```python
from build123d import *

# Parameters (mm, degrees)
SKETCH1_W           = 34.4
SKETCH1_H           = 36
BOSS_EXTRUDE1_DEPTH = 5
SKETCH4_R           = 1.5
CUT_EXTRUDE2_DEPTH  = 5
SKETCH4_3_R         = 1.5
SKETCH4_3_W         = 25.4
SKETCH4_3_H         = 25.4
CUT_EXTRUDE3_DEPTH  = 26.393700006
SKETCH7_W           = 5
SKETCH7_H           = 12
CUT_EXTRUDE4_DEPTH  = 5
SKETCH8_W           = 15
SKETCH8_H           = 3
CUT_EXTRUDE5_DEPTH  = 26.393700006
SKETCH9_W           = 6.4
SKETCH9_H           = 3
CUT_EXTRUDE6_DEPTH  = 26.393700006
SKETCH10_W          = 2
SKETCH10_H          = 3
CUT_EXTRUDE7_DEPTH  = 26.393700006
SKETCH11_W          = 2
SKETCH11_H          = 3
SKETCH11_W_2        = 15
CUT_EXTRUDE8_DEPTH  = 26.393700006
SKETCH12_W          = 5
SKETCH12_H          = 16.7
CUT_EXTRUDE9_DEPTH  = 26.393700006
SKETCH13_W          = 2
SKETCH13_H          = 3
CUT_EXTRUDE10_DEPTH = 26.393700006


with BuildPart() as part:
    # Sketch1 → Boss-Extrude1 (new body)
    with BuildSketch(Plane(origin=(0, 0, 0), x_dir=(1, 0, 0), z_dir=(0, 1, 0))):
        Rectangle(SKETCH1_W, SKETCH1_H)
    extrude(amount=BOSS_EXTRUDE1_DEPTH)

    # Sketch4 → Cut-Extrude2 (cut)
    with BuildSketch(Plane(origin=(0, 5, 0), x_dir=(1, 0, 0), z_dir=(0, 1, 0))):
        with Locations(Location((-12.7, 15.5, 0), (0, 0, 270))):
            Circle(SKETCH4_R)
    extrude(amount=-CUT_EXTRUDE2_DEPTH, mode=Mode.SUBTRACT)

    # Sketch4_3 → Cut-Extrude3 (cut, through all)
    with BuildSketch(Plane(origin=(0, 5, 0), x_dir=(1, 0, 0), z_dir=(0, 1, 0))):
        with Locations(Location((-12.7, 15.5, 0), (0, 0, 270))):
            Circle(SKETCH4_3_R)
        with Locations(Location((7.7, 15.5, 0), (0, 0, 270))):
            Circle(SKETCH4_3_R)
        with Locations(Location((7.7, -15.5, 0), (0, 0, 270))):
            Circle(SKETCH4_3_R)
        with Locations(Location((-12.7, -15.5, 0), (0, 0, 270))):
            Circle(SKETCH4_3_R)
        with Locations((-2.5, 0)):
            Rectangle(SKETCH4_3_W, SKETCH4_3_H)
    extrude(amount=-CUT_EXTRUDE3_DEPTH, mode=Mode.SUBTRACT)

    # Sketch7 → Cut-Extrude4 (cut)
    with BuildSketch(Plane(origin=(0, 5, 0), x_dir=(1, 0, 0), z_dir=(0, 1, 0))):
        with Locations((12.7, -6.7)):
            Rectangle(SKETCH7_W, SKETCH7_H)
    extrude(amount=-CUT_EXTRUDE4_DEPTH, mode=Mode.SUBTRACT)

    # Sketch8 → Cut-Extrude5 (cut, through all)
    with BuildSketch(Plane(origin=(0, 5, 0), x_dir=(1, 0, 0), z_dir=(0, 1, 0))):
        with Locations((-2.7, -16.5)):
            Rectangle(SKETCH8_W, SKETCH8_H)
    extrude(amount=-CUT_EXTRUDE5_DEPTH, mode=Mode.SUBTRACT)

    # Sketch9 → Cut-Extrude6 (cut, through all)
    with BuildSketch(Plane(origin=(0, 5, 0), x_dir=(1, 0, 0), z_dir=(0, 1, 0))):
        with Locations((14, -16.5)):
            Rectangle(SKETCH9_W, SKETCH9_H)
    extrude(amount=-CUT_EXTRUDE6_DEPTH, mode=Mode.SUBTRACT)

    # Sketch10 → Cut-Extrude7 (cut, through all)
    with BuildSketch(Plane(origin=(0, 5, 0), x_dir=(1, 0, 0), z_dir=(0, 1, 0))):
        with Locations((-16.2, -16.5)):
            Rectangle(SKETCH10_W, SKETCH10_H)
    extrude(amount=-CUT_EXTRUDE7_DEPTH, mode=Mode.SUBTRACT)

    # Sketch11 → Cut-Extrude8 (cut, through all)
    with BuildSketch(Plane(origin=(0, 5, 0), x_dir=(1, 0, 0), z_dir=(0, 1, 0))):
        with Locations((-16.2, 16.5)):
            Rectangle(SKETCH11_W, SKETCH11_H)
        with Locations((-2.7, 16.5)):
            Rectangle(SKETCH11_W_2, SKETCH11_H)
    extrude(amount=-CUT_EXTRUDE8_DEPTH, mode=Mode.SUBTRACT)

    # Sketch12 → Cut-Extrude9 (cut, through all)
    with BuildSketch(Plane(origin=(0, 5, 0), x_dir=(1, 0, 0), z_dir=(0, 1, 0))):
        with Locations((14.7, 9.65)):
            Rectangle(SKETCH12_W, SKETCH12_H)
    extrude(amount=-CUT_EXTRUDE9_DEPTH, mode=Mode.SUBTRACT)

    # Sketch13 → Cut-Extrude10 (cut, through all)
    with BuildSketch(Plane(origin=(0, 5, 0), x_dir=(1, 0, 0), z_dir=(0, 1, 0))):
        with Locations((11.2, 16.5)):
            Rectangle(SKETCH13_W, SKETCH13_H)
    extrude(amount=-CUT_EXTRUDE10_DEPTH, mode=Mode.SUBTRACT)


solid = part.part
```
Here's how the part is built. I have some questions about the finished solid (model axes, mm). A direction names the side the tool comes from. Coordinates: 2 decimals unless noted, no trailing zeros. Loops run counter-clockwise (first coordinate to the right, second up) from the corner with the lowest first, then second, coordinate; pieces in that order, holes last. Notation, with made-up numbers: (89.25, 32) - (104.25, 32) arc R22 ccw to (104.25, 47) - close; hole circle Ø1 at (33.5, -21.5). An arc over 180 degrees is marked (long way). Return JSON: item names as keys, results as strings. Group by question number.
Item 1: If we section it at D-D on y = 1.3: State how many separate pieces and enclosed holes the cut face has, and give its area (3 significant figures).
Item 2: Will these pins go through, and if not, where does the flat tip stop? P1, Ø0.9, axis at y = 3, z = 16.5, coming from the -X side; P2, Ø1.5, axis at x = 12.5, y = 2, coming from the +Z side; P3, Ø2.5, axis at y = 3.5, z = 16.5, coming from the +X side; P4, Ø3.5, axis at x = 7.7, z = -15.5, coming from the +Y side.
Item 3: If we section it at B-B on z = -15.5: Write out the boundary of the cut face in (x, y).
Item 4: If we section it at A-A on x = 7.7: Write out the boundary of the cut face in (y, z).
Item 5: I need wall thicknesses on line 1 (X direction, y = 3.85, z = -15.5); line 2 (X direction, y = 1.45, z = 15.5); line 3 (X direction, y = 0.9, z = -6.5). Which ranges of each line are inside material? Lowest first, please. Write a range as from..to.
Item 6: If we section it at C-C on x = -1.5: Write out the boundary of the cut face in (y, z), and give its area (3 significant figures).
Item 7: On a 3-axis mill with a long thin cutter (end or side, diameter ignored), from which of +Z, -Z, +X, -X, +Y, -Y can I reach the whole of each face in a straight line? I mean faces 1 (the face through (10.8, 3, 17)), 2 (the face through (4.8, 3, 17)), 3 (the face through (-10.2, 3, -16)), 4 (the face through (10.2, 3, -6)), 5 (the face through (-16, 3, -15)). Say none if no direction works.
Item 8: We'd pull the mould along Z, two halves only. Please class faces 6 (the face through (-3, 3, -12.7)), 7 (the face through (11, 3, -15)), 8 (the face through (8, 2, 18)): +Z half, -Z half, draft (parallel to the pull), parting line (faces both ways), or undercut.
Calculated:
{
 "1": {"separate pieces": "1", "enclosed holes": "5", "area": "294 mm^2"},
 "2": {"P1": "stops at x = -15.2", "P2": "stops at z = 15", "P3": "stops at x = 10.8", "P4": "stops at y = 5"},
 "3": {"outline": "(-15.2, 0) - (-14.2, 0) - (-14.2, 5) - (-15.2, 5) - close; (-11.2, 0) - (-10.2, 0) - (-10.2, 5) - (-11.2, 5) - close; (4.8, 0) - (6.2, 0) - (6.2, 5) - (4.8, 5) - close; (9.2, 0) - (10.2, 0) - (10.2, 5) - (9.2, 5) - close"},
 "4": {"outline": "(0, -18) - (5, -18) - (5, -17) - (0, -17) - close; (0, -14) - (5, -14) - (5, -12.7) - (0, -12.7) - close; (0, 12.7) - (5, 12.7) - (5, 14) - (0, 14) - close; (0, 17) - (5, 17) - (5, 18) - (0, 18) - close"},
 "5": {"line 1": "x = -15.2..-14.2, -11.2..-10.2, 4.8..6.2, 9.2..10.2", "line 2": "x = -15.2..-14.2, -11.2..-10.2, 4.8..6.2, 9.2..10.8", "line 3": "x = -17.2..-15.2, 10.2..12.2"},
 "6": {"outline": "(0, -15) - (5, -15) - (5, -12.7) - (0, -12.7) - close; (0, 12.7) - (5, 12.7) - (5, 15) - (0, 15) - close", "area": "23.0 mm^2"},
 "7": {"face 1": "+Z, +X, +Y, -Y", "face 2": "+Z, +Y, -Y", "face 3": "-Z, +Y, -Y", "face 4": "+Y, -Y", "face 5": "-Z, -X, +Y, -Y"},
 "8": {"face 6": "undercut", "face 7": "-Z half", "face 8": "+Z half"}
}
